Read the model definition and answer for the solid it produces. Units are mm, in the model's axes. Face numbers are marked on the shaded views. A direction names the side the tool comes from. Round coordinates to 2 decimals unless told otherwise and drop trailing zeros. Write each loop counter-clockwise with the first axis right and the second up, starting at its lowest first coordinate (ties: lowest second). Pieces come first, ordered by that corner, then holes. Notation, with made-up numbers: (-29.5, 32) - (-18.5, 32) arc R23 ccw to (-18.5, 63) - close; hole circle Ø7 at (33.5, 10). An arc over 180 degrees is marked (long way). One line per item, written item: value. Start each with the question number.
(1) Flat-ended cylindrical pins translate along their axes: pin 1 Ø12 at (x, y) = (47, 33.5) entering from +Z (3 decimals); pin 2 Ø5 at (x, y) = (6, 5) entering from +Z; pin 3 Ø6 at (x, z) = (0.5, 24) entering from -Y; pin 4 Ø7.5 at (y, z) = (3.5, 18.5) entering from +X. Find the tip coordinate at first contact, or state that the pin passes through.
(2) A cutting plane is placed at B-B, the plane x = -1.5. Determine the outline of the cut face in (y, z) (1 decimal).
(3) A cutting plane is placed at D-D, the plane x = 23.5. Determine the outline of the cut face in (y, z) (3 decimals), plus the area to 3 significant figures.
(4) The mould has two halves that part along Z. Classify the marked faces 1, 2, 3 and 4: +Z half, -Z half, draft (parallel to the pull), parting line (faces both ways), or undercut.
(5) Find the intervals of material crossed by L1, parallel to Y at x = -16.5, z = 18 (3 decimals); L2, parallel to X at y = 53.5, z = 13.5, in increasing order.
(6) For the marked faces 5, 6 and 7, determine the directions among +Z, -Z, +X, -X, +Y, -Y from which every point of the face is accessible in a straight line to the end or side of a thin tool.
(7) A cutting plane is placed at C-C, the plane y = 42. Determine the outline of the cut face in (x, z) (3 decimals), plus the area to 3 significant figures.
(8) A cutting plane is placed at A-A, the plane y = 5.5. Determine the outline of the cut face in (x, z) (1 decimal), plus the area to 3 significant figures.
from build123d import *

# Parameters (mm, degrees)
SKETCH1_R           = 5.55625
BOSS_EXTRUDE1_DEPTH = 9.525
BOSS_EXTRUDE2_DEPTH = 9.525
SKETCH4_W           = 36.217026874
SKETCH4_H           = 9.525
BOSS_EXTRUDE3_DEPTH = 9.525


with BuildPart() as part:
    # Sketch1 → Boss-Extrude1 (new body)
    with BuildSketch(Plane(origin=(0, 0, 0), x_dir=(1, 0, 0), z_dir=(0, 1, 0))):
        with BuildLine():
            Line((29.36875, 0), (-29.36875, 0))
            Line((-29.36875, 0), (-29.36875, -23.8125))
            ThreePointArc((-29.36875, -23.8125), (-25.649006121, -32.792756121), (-16.66875, -36.5125))
            Line((-16.66875, -36.5125), (16.66875, -36.5125))
            ThreePointArc((16.66875, -36.5125), (25.649006121, -32.792756121), (29.36875, -23.8125))
            Line((29.36875, -23.8125), (29.36875, 0))
        make_face()
        with Locations((-16.66875, -23.8125)):
            Circle(SKETCH1_R, mode=Mode.SUBTRACT)
        with Locations((16.66875, -23.8125)):
            Circle(SKETCH1_R, mode=Mode.SUBTRACT)
    extrude(amount=BOSS_EXTRUDE1_DEPTH)

    # Sketch2 → Boss-Extrude2 (add)
    with BuildSketch(Plane(origin=(0, 0, 0), x_dir=(-1, 0, 0), z_dir=(0, 0, -1))):
        Polygon((-29.36875, 0), (-63.682676038, 53.756755119), (-33.154823962, 73.243244881), (29.36875, 9.525), (29.36875, 0), align=None)
    extrude(amount=-BOSS_EXTRUDE2_DEPTH)

    # Sketch4 → Boss-Extrude3 (add)
    with BuildSketch(Plane(origin=(42.816043465, 67.076310684, 0), x_dir=(0.842914361, -0.538047748, 0), z_dir=(0.538047748, 0.842914361, 0))):
        with Locations((6.646827712, -4.7625)):
            Rectangle(SKETCH4_W, SKETCH4_H)
        with BuildLine():
            Line((-1.290672288, -28.575), (-11.461685725, -28.575))
            ThreePointArc((-11.461685725, -28.575), (6.646827712, -46.683513437), (24.755341149, -28.575))
            Line((24.755341149, -28.575), (14.584327712, -28.575))
            ThreePointArc((14.584327712, -28.575), (6.646827712, -36.5125), (-1.290672288, -28.575))
        make_face()
        with BuildLine():
            Line((24.755341149, -9.525), (-11.461685725, -9.525))
            Line((-11.461685725, -9.525), (-11.461685725, -28.575))
            Line((-11.461685725, -28.575), (-1.290672288, -28.575))
            ThreePointArc((-1.290672288, -28.575), (6.646827712, -20.6375), (14.584327712, -28.575))
            Line((14.584327712, -28.575), (24.755341149, -28.575))
            Line((24.755341149, -28.575), (24.755341149, -9.525))
        make_face()
    extrude(amount=-BOSS_EXTRUDE3_DEPTH)


solid = part.part
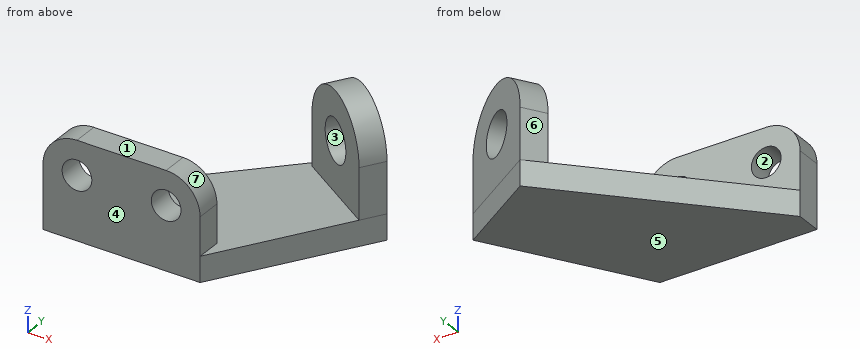
Here are the results:
1. pin 1: z = 9.525
1. pin 2: z = 36.51
1. pin 3: y = 0
1. pin 4: x = 29.37
2. outline: (0, 0) - (37.9, 0) - (37.9, 9.5) - (9.5, 9.5) - (9.5, 36.5) - (0, 36.5) - close
3. outline: (0, 0) - (63.404, 0) - (63.404, 9.525) - (9.525, 9.525) - (9.525, 34.519) - (0, 34.519) - close
3. area: 842 mm²
4. face 1: +Z half
4. face 2: undercut
4. face 3: undercut
4. face 4: draft
5. L1: 0 to 9.525
5. L2: 46.38 to 63.52
6. face 5: -Z, +X, -X, +Y, -Y
6. face 6: +Z, -X, +Y
6. face 7: +Z, +X, -Y
7. outline: (2.497, 0) - (56.178, 0) - (56.178, 9.525) - (2.497, 9.525) - close
7. area: 511 mm²
8. outline: (-29.4, 0) - (32.9, 0) - (32.9, 9.5) - (29.4, 9.5) - (29.4, 23.8) arc R12.7 ccw to (16.7, 36.5) - (-16.7, 36.5) arc R12.7 ccw to (-29.4, 23.8) - close; hole circle Ø11.1 at (-16.7, 23.8); hole circle Ø11.1 at (16.7, 23.8)
8. area: 1,910 mm²
